The listing builds one solid part. Answer for the finished solid, in the listing's coordinates (mm). Face numbers are marked on the shaded views. A direction names the side the tool comes from. Coordinates: 2 decimals unless noted, no trailing zeros. Order: outer loops, then holes, each group sorted by start corner. A loop starts at its lowest first (then second) coordinate and runs counter-clockwise, first axis right, second up.
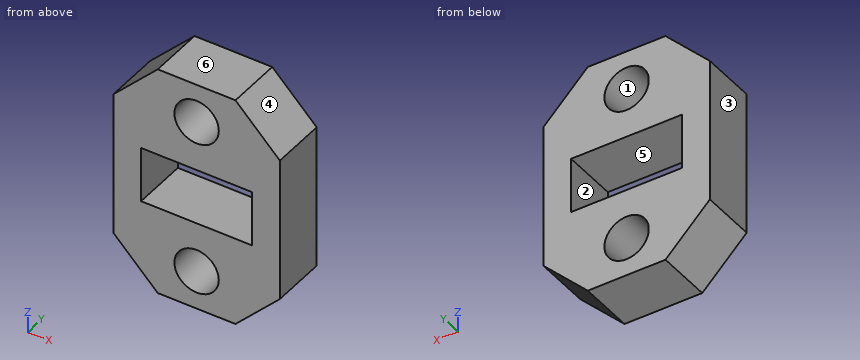
from build123d import *

# Parameters (mm, degrees)
SKETCH1_W           = 15
SKETCH1_H           = 21
BOSS_EXTRUDE1_DEPTH = 5
SKETCH2_R           = 2
SKETCH2_W           = 10
SKETCH2_H           = 5
CUT_EXTRUDE1_DEPTH  = 5
CHAMFER1_SIZE       = 4


with BuildPart() as part:
    # Sketch1 → Boss-Extrude1 (new body)
    with BuildSketch(Plane(origin=(0, 0, 0), x_dir=(1, 0, 0), z_dir=(0, 1, 0))):
        Rectangle(SKETCH1_W, SKETCH1_H)
    extrude(amount=BOSS_EXTRUDE1_DEPTH)

    # Sketch2 → Cut-Extrude1 (cut)
    with BuildSketch(Plane(origin=(0, 5, 0), x_dir=(1, 0, 0), z_dir=(0, 1, 0))):
        with Locations((0, 7)):
            Circle(SKETCH2_R)
        with Locations((0, -7)):
            Circle(SKETCH2_R)
        Rectangle(SKETCH2_W, SKETCH2_H)
    extrude(amount=-CUT_EXTRUDE1_DEPTH, mode=Mode.SUBTRACT)

    # Chamfer1
    chamfer1_edges = [part.edges().sort_by_distance(p)[0] for p in [
        (7.5, 2.5, 10.5),
        (-7.5, 2.5, 10.5),
        (-7.5, 2.5, -10.5),
        (7.5, 2.5, -10.5),
    ]]
    chamfer(chamfer1_edges, length=CHAMFER1_SIZE)


solid = part.part
1) Section B-B (x = 0) is taken. Give the vertices of the cut face in (y, z), then the cut area to 3 significant figures.
2) Determine the mould class of the marked faces 1, 2, 3 and 4 for opening direction Z: released by +Z, released by -Z, zero draft, split by the parting line, or undercut.
3) Section C-C (y = 3.7) is taken. Give the vertices of the cut face in (x, z), then the cut area to 3 significant figures.
4) Section A-A (z = -7) is taken. Give the vertices of the cut face in (x, y), then the cut area to 3 significant figures.
5) Section D-D (z = -1) is taken. Give the vertices of the cut face in (x, y), then the cut area to 3 significant figures.
6) A tool of negligible diameter and unlimited length cuts with its end or side. For the marked faces 5 and 6, from which of +Z, -Z, +X, -X, +Y, -Y can it reach the whole face along a straight path? Write none if from no direction.
7) Consider L1, parallel to Z at x = 0, y = 3.7; L2, parallel to Z at x = -3.25, y = 3.35; L3, parallel to X at y = 2.75, z = 1.75. Determine where each line is inside the solid, lowest interval first.
Filled sheet:
1. outline: (0, -10.5) - (5, -10.5) - (5, -9) - (0, -9) - close; (0, -5) - (5, -5) - (5, -2.5) - (0, -2.5) - close; (0, 2.5) - (5, 2.5) - (5, 5) - (0, 5) - close; (0, 9) - (5, 9) - (5, 10.5) - (0, 10.5) - close
1. area: 40.0 mm2
2. face 1: undercut
2. face 2: undercut
2. face 3: zero draft
2. face 4: released by +Z
3. outline: (-7.5, -6.5) - (-3.5, -10.5) - (3.5, -10.5) - (7.5, -6.5) - (7.5, 6.5) - (3.5, 10.5) - (-3.5, 10.5) - (-7.5, 6.5) - close; hole (-5, -2.5) - (5, -2.5) - (5, 2.5) - (-5, 2.5) - close; hole circle Ø4 at (0, -7); hole circle Ø4 at (0, 7)
3. area: 208 mm2
4. outline: (-7, 0) - (-2, 0) - (-2, 5) - (-7, 5) - close; (2, 0) - (7, 0) - (7, 5) - (2, 5) - close
4. area: 50.0 mm2
5. outline: (-7.5, 0) - (-5, 0) - (-5, 5) - (-7.5, 5) - close; (5, 0) - (7.5, 0) - (7.5, 5) - (5, 5) - close
5. area: 25.0 mm2
6. face 5: +Y, -Y
6. face 6: +Z, +X, -X, +Y, -Y
7. L1: z = -10.5 to -9, -5 to -2.5, 2.5 to 5, 9 to 10.5
7. L2: z = -10.5 to -2.5, 2.5 to 10.5
7. L3: x = -7.5 to -5, 5 to 7.5
